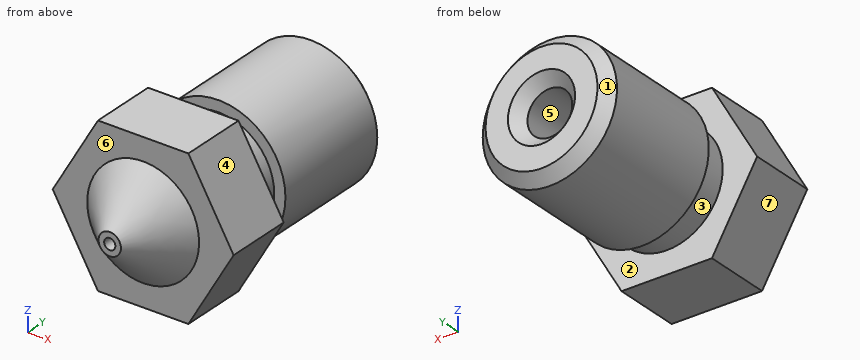
from build123d import *

# Parameters (mm, degrees)
BOSS_EXTRUDE1_DEPTH = 3
CHAMFER1_SIZE       = 0.5


with BuildPart() as part:
    # Sketch1 → Boss-Extrude1 (new body)
    with BuildSketch(Plane.XZ):
        Polygon((-2.020725942, 3.5), (-4.041451884, 0), (-2.020725942, -3.5), (2.020725942, -3.5), (4.041451884, 0), (2.020725942, 3.5), align=None)
    extrude(amount=-BOSS_EXTRUDE1_DEPTH)

    # Sketch2 → Revolve1 (revolve)
    with BuildSketch(Plane(origin=(0, 0, 0), x_dir=(-1, 0, 0), z_dir=(0, 0, -1))):
        Polygon((-2.5, 3), (0, 3), (0, 10.5), (-3, 10.5), (-3, 4.5), (-2.5, 4.5), align=None)
    revolve(axis=Axis((0, 3, 0), (0, 1, 0)))

    # Sketch3 → Revolve2 (revolve)
    with BuildSketch(Plane.XY):
        Polygon((2.5, 0), (0, 0), (0, -2), (0.5, -2), align=None)
    revolve(axis=Axis((0, 0, 0), (0, -1, 0)))

    # Sketch4 → Cut-Revolve1 (revolve, cut)
    with BuildSketch(Plane(origin=(0, 0, 0), x_dir=(-1, 0, 0), z_dir=(0, 0, -1))):
        Polygon((-0.25, -2), (0, -2), (0, 10.5), (-1, 10.5), (-1, 0), (-0.75, -0.227272727), (-0.75, -0.7), (-0.25, -1.2), align=None)
    revolve(axis=Axis((0, -2, 0), (0, 1, 0)), mode=Mode.SUBTRACT)

    # Chamfer1
    chamfer1_edges = [part.edges().sort_by_distance(p)[0] for p in [
        (-3, 10.5, 0),
        (-1, 10.5, 0),
    ]]
    chamfer(chamfer1_edges, length=CHAMFER1_SIZE)


solid = part.part
Here's how the part is built. I have some questions about the finished solid (model axes, mm). Face numbers are marked on the shaded views. A direction names the side the tool comes from. Coordinates: 2 decimals unless noted, no trailing zeros. Order: outer loops, then holes, each group sorted by start corner. A loop starts at its lowest first (then second) coordinate and runs counter-clockwise, first axis right, second up. Notation, with made-up numbers: M 76.5,-8.5 L 80.5,-8.5 A28 ccw 80.5,22.5 Z; hole C 84,22 d7. An arc over 180 degrees is marked long. Answer as CSV lines item,"result". Start each with the question number.
1. I want a section at A-A, the plane y = 1.5. Write out the boundary of the cut face in (x, z), and give its area (3 significant figures).
2. I want a section at D-D, the plane x = 3.5. Write out the boundary of the cut face in (y, z), and give its area (3 significant figures).
3. I want a section at C-C, the plane y = 7.75. Write out the boundary of the cut face in (x, z).
4. We'd pull the mould along Y, two halves only. Please class the marked faces 1, 2, 3 and 4: released by +Y, released by -Y, zero draft, split by the parting line, or undercut.
5. For pin 1 (1.4 mm diameter, centred on x = 0, z = 0, fed in from +Y); pin 2 (3.5 mm diameter, centred on x = 1, z = 0.5, fed in from +Y); pin 3 (4 mm diameter, centred on y = 6.5, z = -0.5, fed in from -X); pin 4 (1 mm diameter, centred on x = -3, z = -2, fed in from -Y), each with a flat end and sliding along its axis, tell me the tip position at first contact or that it passes through.
6. I need wall thicknesses on line 1 (X direction, y = 3.5, z = 0); line 2 (Z direction, x = 0, y = 2.5); line 3 (Z direction, x = 0, y = 7). Which ranges of each line are inside material? Lowest first, please. Write a range as [from, to].
7. On a 3-axis mill with a long thin cutter (end or side, diameter ignored), from which of +Z, -Z, +X, -X, +Y, -Y can I reach the whole of each face in a straight line? I mean the marked faces 5, 6 and 7. Say none if no direction works.
Recorded:
1,outline,"M -4.04,0 L -2.02,-3.5 L 2.02,-3.5 L 4.04,0 L 2.02,3.5 L -2.02,3.5 Z; hole C 0,0 d2"
1,area,"39.3 mm2"
2,outline,"M 0,-0.94 L 3,-0.94 L 3,0.94 L 0,0.94 Z"
2,area,"5.63 mm2"
3,outline,"C 0,0 d6; hole C 0,0 d2"
4,face 1,"released by +Y"
4,face 2,"undercut"
4,face 3,"undercut"
4,face 4,"zero draft"
5,pin 1,"stops at y = -0.75"
5,pin 2,"stops at y = 10.5"
5,pin 3,"stops at x = -3"
5,pin 4,"stops at y = 0"
6,line 1,"x = [-2.5, -1], [1, 2.5]"
6,line 2,"z = [-3.5, -1], [1, 3.5]"
6,line 3,"z = [-3, -1], [1, 3]"
7,face 5,"+Y"
7,face 6,"-Y"
7,face 7,"-Z, -X, +Y, -Y"
